from build123d import *

# Parameters (mm, degrees)
SKETCH_1_W          = 57
SKETCH_1_H          = 40
EXTRUDE_1_DEPTH     = 45
SKETCH_5_R          = 13
CUT_EXTRUDE_1_DEPTH = 17.8
CUT_EXTRUDE_2_DEPTH = 36.2
SKETCH_7_R          = 13
CUT_EXTRUDE_3_DEPTH = 31.1
CUT_EXTRUDE_5_DEPTH = 83.909589313
SKETCH_12_R         = 2
CUT_EXTRUDE_6_DEPTH = 8
SKETCH_13_R         = 1.5
CUT_EXTRUDE_7_DEPTH = 76.325958341
CUT_EXTRUDE_9_DEPTH = 94
SKETCH_16_W         = 40
SKETCH_16_H         = 39
SKETCH_16_R         = 2
SKETCH_16_R_2       = 13
EXTRUDE_2_DEPTH     = 1.5
EXTRUDE_START       = 1.5
SKETCH_17_W         = 34.7
SKETCH_17_H         = 40
SKETCH_17_R         = 1.5
EXTRUDE_3_DEPTH     = 1.5
SKETCH_18_W         = 34.7
SKETCH_18_H         = 40
SKETCH_18_R         = 1.5
EXTRUDE_4_DEPTH     = 1.5
EXTRUDE_START_2     = 1
SKETCH_20_W         = 40
SKETCH_20_H         = 37.911419384
SKETCH_20_R         = 13
EXTRUDE_6_DEPTH     = 1


with BuildPart() as part:
    # 草图1 → 凸台-拉伸1 (new body)
    with BuildSketch(Plane(origin=(0, 0, 0), x_dir=(1, 0, 0), z_dir=(0, 1, 0))):
        with Locations((-28.5, 0)):
            Rectangle(SKETCH_1_W, SKETCH_1_H)
    extrude(amount=EXTRUDE_1_DEPTH)

    # 草图5 → 切除-拉伸1 (cut)
    with BuildSketch(Plane(origin=(0, 0, 0), x_dir=(0, 0, -1), z_dir=(1, 0, 0))):
        with Locations((0, 22.5)):
            Circle(SKETCH_5_R)
    extrude(amount=-CUT_EXTRUDE_1_DEPTH, mode=Mode.SUBTRACT)

    # 草图6 → 切除-拉伸2 (cut)
    with BuildSketch(Plane(origin=(-17.8, 0, 0), x_dir=(0, 0, -1), z_dir=(1, 0, 0))):
        Polygon((-22, 25), (-22, 3), (22, 3), (22, 25), (22, 42), (-22, 42), align=None)
    extrude(amount=-CUT_EXTRUDE_2_DEPTH, mode=Mode.SUBTRACT)

    # 草图7 → 切除-拉伸3 (cut)
    with BuildSketch(Plane(origin=(-54, 0, 0), x_dir=(0, 0, -1), z_dir=(1, 0, 0))):
        with Locations((0, 22.5)):
            Circle(SKETCH_7_R)
    extrude(amount=-CUT_EXTRUDE_3_DEPTH, mode=Mode.SUBTRACT)

    # 草图10 → 切除-拉伸5 (cut, through all)
    with BuildSketch(Plane.XY.offset(20)):
        Polygon((-15, 45), (0, 40.126204557), (0, 45), align=None)
        Polygon((0, 0), (-15, 0), (0, 4.873795443), align=None)
    extrude(amount=-CUT_EXTRUDE_5_DEPTH, mode=Mode.SUBTRACT)

    # 草图12 → 切除-拉伸6 (cut)
    with BuildSketch(Plane.ZY.offset(57)):
        with Locations((-12.374368671, 34.874368671)):
            Circle(SKETCH_12_R)
        with Locations((12.374368671, 34.874368671)):
            Circle(SKETCH_12_R)
        with Locations((12.374368671, 10.125631329)):
            Circle(SKETCH_12_R)
        with Locations((-12.374368671, 10.125631329)):
            Circle(SKETCH_12_R)
    extrude(amount=-CUT_EXTRUDE_6_DEPTH, mode=Mode.SUBTRACT)

    # 草图13 → 切除-拉伸7 (cut, through all)
    with BuildSketch(Plane(origin=(0, 45, 0), x_dir=(1, 0, 0), z_dir=(0, 1, 0))):
        with Locations(Location((-45, 15, 0), (0, 0, 270))):
            Circle(SKETCH_13_R)
        with Locations(Location((-27, 15, 0), (0, 0, 270))):
            Circle(SKETCH_13_R)
        with Locations(Location((-27, -15, 0), (0, 0, 270))):
            Circle(SKETCH_13_R)
        with Locations(Location((-45, -15, 0), (0, 0, 270))):
            Circle(SKETCH_13_R)
    extrude(amount=-CUT_EXTRUDE_7_DEPTH, mode=Mode.SUBTRACT)

    # 草图15 → 切除-拉伸9 (cut)
    with BuildSketch(Plane.XY.offset(20)):
        Polygon((-13.8, 41.455709692), (-4, 38.271496669), (-4, 6.728503331), (-13.8, 3.544290308), align=None)
    extrude(amount=-CUT_EXTRUDE_9_DEPTH, mode=Mode.SUBTRACT)

    # 草图16 → 凸台-拉伸2 (add)
    with BuildSketch(Plane(origin=(-54, 0, 0), x_dir=(0, 0, -1), z_dir=(1, 0, 0))):
        with Locations((0, 22.5)):
            Rectangle(SKETCH_16_W, SKETCH_16_H)
        with Locations(Location((-12.374368671, 10.125631329, 0), (0, 0, 180))):
            Circle(SKETCH_16_R, mode=Mode.SUBTRACT)
        with Locations(Location((12.374368671, 10.125631329, 0), (0, 0, 180))):
            Circle(SKETCH_16_R, mode=Mode.SUBTRACT)
        with Locations((0, 22.5)):
            Circle(SKETCH_16_R_2, mode=Mode.SUBTRACT)
        with Locations(Location((12.374368671, 34.874368671, 0), (0, 0, 180))):
            Circle(SKETCH_16_R, mode=Mode.SUBTRACT)
        with Locations(Location((-12.374368671, 34.874368671, 0), (0, 0, 180))):
            Circle(SKETCH_16_R, mode=Mode.SUBTRACT)
    extrude(amount=EXTRUDE_2_DEPTH)

    # 草图17 → 凸台-拉伸3 (add)
    with BuildSketch(Plane(origin=(0, 3, 0), x_dir=(1, 0, 0), z_dir=(0, 1, 0)).offset(EXTRUDE_START)):
        with Locations((-35.15, 0)):
            Rectangle(SKETCH_17_W, SKETCH_17_H)
        with Locations(Location((-45, -15, 0), (0, 0, 270))):
            Circle(SKETCH_17_R, mode=Mode.SUBTRACT)
        with Locations(Location((-27, -15, 0), (0, 0, 270))):
            Circle(SKETCH_17_R, mode=Mode.SUBTRACT)
        with Locations(Location((-27, 15, 0), (0, 0, 270))):
            Circle(SKETCH_17_R, mode=Mode.SUBTRACT)
        with Locations(Location((-45, 15, 0), (0, 0, 270))):
            Circle(SKETCH_17_R, mode=Mode.SUBTRACT)
    extrude(amount=-EXTRUDE_3_DEPTH)

    # 草图18 → 凸台-拉伸4 (add)
    with BuildSketch(Plane.XZ.offset(-42)):
        with Locations((-35.15, 0)):
            Rectangle(SKETCH_18_W, SKETCH_18_H)
        with Locations(Location((-45, -15, 0), (0, 0, 90))):
            Circle(SKETCH_18_R, mode=Mode.SUBTRACT)
        with Locations(Location((-27, -15, 0), (0, 0, 90))):
            Circle(SKETCH_18_R, mode=Mode.SUBTRACT)
        with Locations(Location((-27, 15, 0), (0, 0, 90))):
            Circle(SKETCH_18_R, mode=Mode.SUBTRACT)
        with Locations(Location((-45, 15, 0), (0, 0, 90))):
            Circle(SKETCH_18_R, mode=Mode.SUBTRACT)
    extrude(amount=EXTRUDE_4_DEPTH)

    # 草图20 → 凸台-拉伸6 (add)
    with BuildSketch(Plane(origin=(-13.8, 0, 0), x_dir=(0, 0, -1), z_dir=(1, 0, 0)).offset(EXTRUDE_START_2)):
        with Locations((0, 22.5)):
            Rectangle(SKETCH_20_W, SKETCH_20_H)
        with Locations((0, 22.5)):
            Circle(SKETCH_20_R, mode=Mode.SUBTRACT)
    extrude(amount=-EXTRUDE_6_DEPTH)


solid = part.part
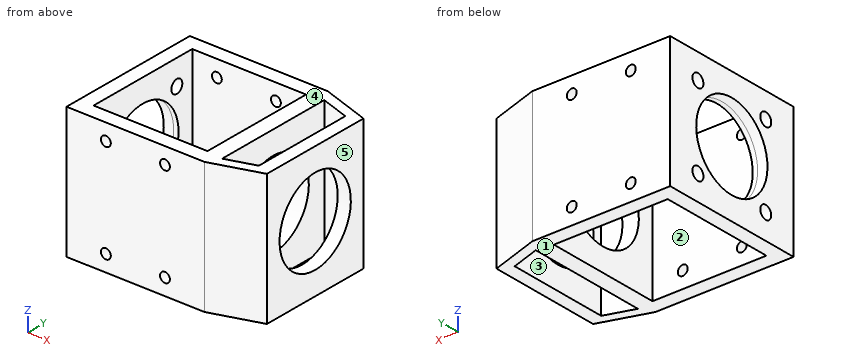
Geometry: final body of the model. Coordinates: model frame, mm. Face numbers are marked on the shaded views. A direction names the side the tool comes from. Give positions to 0.01 mm unless a question says otherwise; leave off trailing zeros. Order: outer loops, then holes, each group sorted by start corner. A loop starts at its lowest first (then second) coordinate and runs counter-clockwise, first axis right, second up. Notation, with made-up numbers: (70.25, 38.25) - (88.25, 38.25) arc R28 cw to (88.25, 60.25) - close; hole circle Ø6 at (43.25, -21.75). An arc over 180 degrees is marked (long way). Use CSV: the item, a comma, the result in double quotes.
1. Section query A-A (x = -35.5). Output: boundary loops of the cut face in (y, z), plus the area to 3 significant figures.
Answers below:
outline,"(0, -20) - (4.5, -20) - (4.5, 20) - (0, 20) - close; (40.5, -20) - (45, -20) - (45, 20) - (40.5, 20) - close"
area,"360 mm2"
2. Access query for the marked faces 1 and 2. Directions: +Z, -Z, +X, -X, +Y, -Y. A direction counts if a zero-diameter tool reaches every point of the face in a straight line with its end or side. Return the directions, or none.
Answers below:
face 1,"-Z, +X, -X, +Y, -Y"
face 2,"+Z, -Z"
3. Section query D-D (z = -7). Output: boundary loops of the cut face in (x, y).
Answers below:
outline,"(-57, 0) - (-15, 0) - (0, 4.87) - (0, 11.55) - (-4, 11.55) - (-4, 6.73) - (-12.8, 3.87) - (-12.8, 11.55) - (-17.8, 11.55) - (-17.8, 4.5) - (-52.5, 4.5) - (-52.5, 11.55) - (-57, 11.55) - close; (-57, 33.45) - (-52.5, 33.45) - (-52.5, 40.5) - (-17.8, 40.5) - (-17.8, 33.45) - (-12.8, 33.45) - (-12.8, 41.13) - (-4, 38.27) - (-4, 33.45) - (0, 33.45) - (0, 40.13) - (-15, 45) - (-57, 45) - close"
4. Mould query, pull axis X, two halves, no side actions, for the marked faces 3, 4 and 5. Classes: +X half, -X half, draft (parallel to the pull), parting line (faces both ways), or undercut.
Answers below:
face 3,"undercut"
face 4,"draft"
face 5,"+X half"
5. Contact query for flat-ended pins moving along their axis: pin 1 (2 mm diameter, centred on y = 34, z = -14.5, fed in from +X); pin 2 (10 mm diameter, centred on x = -8, z = 6.5, fed in from +Y); pin 3 (3 mm diameter, centred on y = 34.87, z = 12.37, fed in from -X). Output: stop coordinate, or through.
Answers below:
pin 1,"x = 0"
pin 2,"y = 44.35"
pin 3,"x = -17.8"
6. Section query B-B (y = 22.5). Output: boundary loops of the cut face in (x, z), plus the area to 3 significant figures.
Answers below:
outline,"(-57, -20) - (-52.5, -20) - (-52.5, -13) - (-57, -13) - close; (-57, 13) - (-52.5, 13) - (-52.5, 20) - (-57, 20) - close; (-17.8, -20) - (-12.8, -20) - (-12.8, -13) - (-17.8, -13) - close; (-17.8, 13) - (-12.8, 13) - (-12.8, 20) - (-17.8, 20) - close; (-4, -20) - (0, -20) - (0, -13) - (-4, -13) - close; (-4, 13) - (0, 13) - (0, 20) - (-4, 20) - close"
area,"189 mm2"
7. Material intervals for line 1 along X through (y, z) = (26, 15.5); line 2 along Z through (x, y) = (-27, 42.35); line 3 along Y through (x, z) = (-47.5, -7), sorted ascending. Write a range as from..to.
Answers below:
line 1,"-57..-52.5, -17.8..-12.8, -4..0"
line 2,"-20..-16.5, -13.5..13.5, 16.5..20"
line 3,"0..4.5, 40.5..45"
8. Section query C-C (x = -27). Output: boundary loops of the cut face in (y, z), plus the area to 3 significant figures.
Answers below:
outline,"(0, -20) - (4.5, -20) - (4.5, -16.5) - (0, -16.5) - close; (0, -13.5) - (4.5, -13.5) - (4.5, 13.5) - (0, 13.5) - close; (0, 16.5) - (4.5, 16.5) - (4.5, 20) - (0, 20) - close; (40.5, -20) - (45, -20) - (45, -16.5) - (40.5, -16.5) - close; (40.5, -13.5) - (45, -13.5) - (45, 13.5) - (40.5, 13.5) - close; (40.5, 16.5) - (45, 16.5) - (45, 20) - (40.5, 20) - close"
area,"306 mm2"
